The model under review builds one solid part; all positions refer to its coordinate system, in mm. Face numbers are marked on the shaded views. A direction names the side the tool comes from. Coordinates: 2 decimals unless noted, no trailing zeros. Loops run counter-clockwise (first coordinate to the right, second up) from the corner with the lowest first, then second, coordinate; pieces in that order, holes last. Notation, with made-up numbers: (11, 2.5) - (36, 2.5) arc R27 ccw to (36, 40.5) - close; hole circle Ø9 at (23, -2). An arc over 180 degrees is marked (long way). Answer in a Markdown table with one row per item. Add a question column.
(1) We need section C-C on z = 1.7. Give the number of separate pieces and of enclosed holes in the cut face, plus the area to 3 significant figures.
(2) We need section A-A on y = 7. Write out the cut boundary in (x, z), plus the area to 3 significant figures.
(3) We need section B-B on x = 8.5. Write out the cut boundary in (y, z), plus the area to 3 significant figures.
(4) We need section D-D on x = -21. Write out the cut boundary in (y, z), plus the area to 3 significant figures.
(5) Mouldability with a two-part tool opening along X and no side actions: class the marked faces 3, 4, 5 and 6 as +X half, -X half, draft (parallel to the pull), parting line (faces both ways), or undercut.
(6) For P1, Ø0.8, axis at y = 11, z = 1.5, coming from the +X side; P2, Ø0.8, axis at x = 11, z = 1.5, coming from the -Y side, all flat-tipped, find the tip position at first contact; note any pin that passes through.
(7) Machinability: for the marked faces 1 and 2, which of the approach directions +Z, -Z, +X, -X, +Y, -Y give a long, thin tool a straight path to every point of the face, cutting with its end or side? Answer none if there is none.
(8) For line 1 along X through (y, z) = (17.5, 2.25); line 2 along X through (y, z) = (-3, 1); line 3 along Y through (x, z) = (7, 0.4), list the stretches that pass through material, from the lowest coordinate up.
from build123d import *

# Parameters (mm, degrees)
F0_R     = 2.5
F1_DEPTH = 2.5


with BuildPart() as f1:
    # F0 (on Top) → F1 (new body)
    with BuildSketch(Plane.XY):
        with BuildLine():
            Line((-3.200922, 22.332565), (-25.390672, 3.841106))
            ThreePointArc((-25.390672, 3.841106), (-21.653839, 4.971197), (-18.243719, 3.070641))
            ThreePointArc((-18.243719, 3.070641), (-18.63819, 4.44548), (-17.972234, 5.711296))
            Line((-17.972234, 5.711296), (-14.210711, 8.909378))
            ThreePointArc((-14.210711, 8.909378), (-13.407208, 9.207037), (-12.600804, 8.917329))
            Line((-12.600804, 8.917329), (-6.052341, 3.460277))
            ThreePointArc((-6.052341, 3.460277), (-5.677232, 2.074468), (-6.852572, 1.25))
            Line((-6.852572, 1.25), (-16.461531, 1.25))
            ThreePointArc((-16.461531, 1.25), (-17.146184, 1.454175), (-17.607175, 2))
            ThreePointArc((-17.607175, 2), (-17.295219, 1.021548), (-17.18975, 0))
            ThreePointArc((-17.18975, 0), (-17.295219, -1.021548), (-17.607175, -2))
            ThreePointArc((-17.607175, -2), (-17.146184, -1.454175), (-16.461531, -1.25))
            Line((-16.461531, -1.25), (-6.852572, -1.25))
            ThreePointArc((-6.852572, -1.25), (-5.677232, -2.074468), (-6.052341, -3.460277))
            Line((-6.052341, -3.460277), (-12.600804, -8.917329))
            ThreePointArc((-12.600804, -8.917329), (-13.407208, -9.207037), (-14.210711, -8.909378))
            Line((-14.210711, -8.909378), (-17.972234, -5.711296))
            ThreePointArc((-17.972234, -5.711296), (-18.63819, -4.44548), (-18.243719, -3.070641))
            ThreePointArc((-18.243719, -3.070641), (-21.653839, -4.971197), (-25.390672, -3.841106))
            Line((-25.390672, -3.841106), (-3.200922, -22.332565))
            ThreePointArc((-3.200922, -22.332565), (0, -23.491459), (3.200922, -22.332565))
            Line((3.200922, -22.332565), (25.390672, -3.841106))
            ThreePointArc((25.390672, -3.841106), (21.653839, -4.971197), (18.243719, -3.070641))
            ThreePointArc((18.243719, -3.070641), (18.63819, -4.44548), (17.972234, -5.711296))
            Line((17.972234, -5.711296), (14.210711, -8.909378))
            ThreePointArc((14.210711, -8.909378), (13.407208, -9.207037), (12.600804, -8.917329))
            Line((12.600804, -8.917329), (6.052341, -3.460277))
            ThreePointArc((6.052341, -3.460277), (5.677232, -2.074468), (6.852572, -1.25))
            Line((6.852572, -1.25), (16.461531, -1.25))
            ThreePointArc((16.461531, -1.25), (17.146184, -1.454175), (17.607175, -2))
            ThreePointArc((17.607175, -2), (17.18975, 0), (17.607175, 2))
            ThreePointArc((17.607175, 2), (17.146184, 1.454175), (16.461531, 1.25))
            Line((16.461531, 1.25), (6.852572, 1.25))
            ThreePointArc((6.852572, 1.25), (5.677232, 2.074468), (6.052341, 3.460277))
            Line((6.052341, 3.460277), (12.600804, 8.917329))
            ThreePointArc((12.600804, 8.917329), (13.407208, 9.207037), (14.210711, 8.909378))
            Line((14.210711, 8.909378), (17.972234, 5.711296))
            ThreePointArc((17.972234, 5.711296), (18.63819, 4.44548), (18.243719, 3.070641))
            ThreePointArc((18.243719, 3.070641), (21.653839, 4.971197), (25.390672, 3.841106))
            Line((25.390672, 3.841106), (3.200922, 22.332565))
            ThreePointArc((3.200922, 22.332565), (0, 23.491459), (-3.200922, 22.332565))
        make_face()
        with BuildLine():
            Line((-10.259876, -10.363764), (-3.309676, -4.454638))
            ThreePointArc((-3.309676, -4.454638), (-1.975403, -4.272372), (-1.25, -5.406964))
            Line((-1.25, -5.406964), (-1.25, -17.225215))
            ThreePointArc((-1.25, -17.225215), (-1.975403, -18.359806), (-3.309676, -18.177541))
            Line((-3.309676, -18.177541), (-10.259876, -12.268415))
            ThreePointArc((-10.259876, -12.268415), (-10.7002, -11.316089), (-10.259876, -10.363764))
        make_face(mode=Mode.SUBTRACT)
        with BuildLine():
            ThreePointArc((1.25, -5.406964), (1.975403, -4.272372), (3.309676, -4.454638))
            Line((3.309676, -4.454638), (10.259876, -10.363764))
            ThreePointArc((10.259876, -10.363764), (10.7002, -11.316089), (10.259876, -12.268415))
            Line((10.259876, -12.268415), (3.309676, -18.177541))
            ThreePointArc((3.309676, -18.177541), (1.975403, -18.359806), (1.25, -17.225215))
            Line((1.25, -17.225215), (1.25, -5.406964))
        make_face(mode=Mode.SUBTRACT)
        with BuildLine():
            Line((-1.25, 17.225215), (-1.25, 5.406964))
            ThreePointArc((-1.25, 5.406964), (-1.975403, 4.272372), (-3.309676, 4.454638))
            Line((-3.309676, 4.454638), (-10.259876, 10.363764))
            ThreePointArc((-10.259876, 10.363764), (-10.7002, 11.316089), (-10.259876, 12.268415))
            Line((-10.259876, 12.268415), (-3.309676, 18.177541))
            ThreePointArc((-3.309676, 18.177541), (-1.975403, 18.359806), (-1.25, 17.225215))
        make_face(mode=Mode.SUBTRACT)
        with BuildLine():
            ThreePointArc((3.309676, 4.454638), (1.975403, 4.272372), (1.25, 5.406964))
            Line((1.25, 5.406964), (1.25, 17.225215))
            ThreePointArc((1.25, 17.225215), (1.975403, 18.359806), (3.309676, 18.177541))
            Line((3.309676, 18.177541), (10.259876, 12.268415))
            ThreePointArc((10.259876, 12.268415), (10.7002, 11.316089), (10.259876, 10.363764))
            Line((10.259876, 10.363764), (3.309676, 4.454638))
        make_face(mode=Mode.SUBTRACT)
        with BuildLine():
            ThreePointArc((-18.243719, 3.070641), (-21.653839, 4.971197), (-25.390672, 3.841106))
            ThreePointArc((-25.390672, 3.841106), (-27.18975, 0), (-25.390672, -3.841106))
            ThreePointArc((-25.390672, -3.841106), (-21.653839, -4.971197), (-18.243719, -3.070641))
            ThreePointArc((-18.243719, -3.070641), (-17.891977, -2.55522), (-17.607175, -2))
            ThreePointArc((-17.607175, -2), (-17.295219, -1.021548), (-17.18975, 0))
            ThreePointArc((-17.18975, 0), (-17.295219, 1.021548), (-17.607175, 2))
            ThreePointArc((-17.607175, 2), (-17.891977, 2.55522), (-18.243719, 3.070641))
        make_face()
        with Locations((-22.18975, 0)):
            Circle(F0_R, mode=Mode.SUBTRACT)
        with Locations((-22.18975, 0)):
            Circle(F0_R)
        with BuildLine():
            ThreePointArc((27.18975, 0), (26.717697, 2.120777), (25.390672, 3.841106))
            ThreePointArc((25.390672, 3.841106), (21.653839, 4.971197), (18.243719, 3.070641))
            ThreePointArc((18.243719, 3.070641), (17.891977, 2.55522), (17.607175, 2))
            ThreePointArc((17.607175, 2), (17.18975, 0), (17.607175, -2))
            ThreePointArc((17.607175, -2), (17.891977, -2.55522), (18.243719, -3.070641))
            ThreePointArc((18.243719, -3.070641), (21.653839, -4.971197), (25.390672, -3.841106))
            ThreePointArc((25.390672, -3.841106), (26.717697, -2.120777), (27.18975, 0))
        make_face()
        with Locations((22.18975, 0)):
            Circle(F0_R, mode=Mode.SUBTRACT)
        with Locations((22.18975, 0)):
            Circle(F0_R)
    extrude(amount=F1_DEPTH)


solid = f1.part
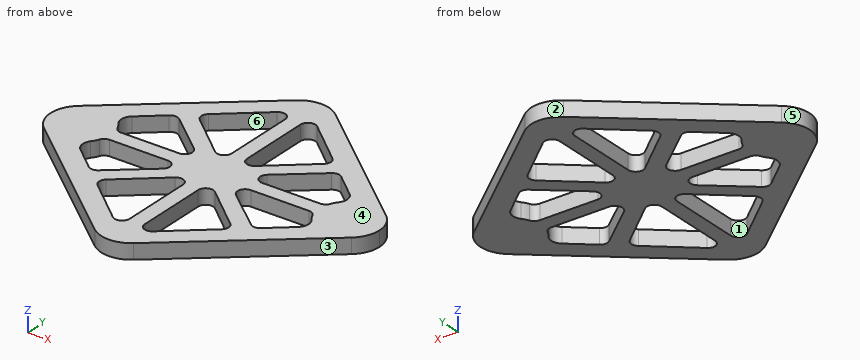
Outcome:
| question | item | result |
|---|---|---|
| 1 | separate pieces | 1 |
| 1 | enclosed holes | 8 |
| 1 | area | 866 mm² |
| 2 | outline | (-21.6, 0) - (-16.46, 0) - (-16.46, 2.5) - (-21.6, 2.5) - close; (-10.3, 0) - (-6.3, 0) - (-6.3, 2.5) - (-10.3, 2.5) - close; (-1.25, 0) - (1.25, 0) - (1.25, 2.5) - (-1.25, 2.5) - close; (6.3, 0) - (10.3, 0) - (10.3, 2.5) - (6.3, 2.5) - close; (16.46, 0) - (21.6, 0) - (21.6, 2.5) - (16.46, 2.5) - close |
| 2 | area | 52.0 mm² |
| 3 | outline | (-17.92, 0) - (-13.76, 0) - (-13.76, 2.5) - (-17.92, 2.5) - close; (-8.87, 0) - (-5.5, 0) - (-5.5, 2.5) - (-8.87, 2.5) - close; (-1.25, 0) - (1.25, 0) - (1.25, 2.5) - (-1.25, 2.5) - close; (5.5, 0) - (8.87, 0) - (8.87, 2.5) - (5.5, 2.5) - close; (13.76, 0) - (17.92, 0) - (17.92, 2.5) - (13.76, 2.5) - close |
| 3 | area | 43.8 mm² |
| 4 | outline | (-7.5, 0) - (7.5, 0) - (7.5, 2.5) - (-7.5, 2.5) - close |
| 4 | area | 37.5 mm² |
| 5 | face 3 | +X half |
| 5 | face 4 | draft |
| 5 | face 5 | -X half |
| 5 | face 6 | undercut |
| 6 | P1 | x = 17.28 |
| 6 | P2 | y = -16.17 |
| 7 | face 1 | +Z, -Z |
| 7 | face 2 | +Z, -Z, +Y |
| 8 | line 1 | -9 to -4.11, -1.28 to 1.28, 4.11 to 9 |
| 8 | line 2 | -26.19 to -18.19, -5.71 to 5.71, 18.19 to 26.19 |
| 8 | line 3 | -19.17 to -15.04, -7.59 to -4.25, -1.25 to 1.25, 4.25 to 7.59, 15.04 to 19.17 |
